Can you work these out from the model? Positions are in its coordinate system, mm. Coordinates: 2 decimals unless noted, no trailing zeros. Loops run counter-clockwise (first coordinate to the right, second up) from the corner with the lowest first, then second, coordinate; pieces in that order, holes last. Notation, with made-up numbers: M 37.25,40 L 60.25,40 A24 cw 60.25,55 Z; hole C -29.75,-24 d7. An arc over 180 degrees is marked long. Return JSON: item names as keys, results as strings. Group by question number.
Autodesk Inventor part; units mm, degrees
ref_plane "YZ Plane" through (0, 0, 0) normal (1, 0, 0) x (0, 1, 0)
ref_plane "XZ Plane" through (0, 0, 0) normal (0, 1, 0) x (-1, 0, 0)
ref_plane "XY Plane" through (0, 0, 0) normal (0, 0, 1) x (1, 0, 0)
sketch "Sketch1" plane through (0, 0, 0) normal (0, 0, 1) x (1, 0, 0)
  line L0 (-88.9, 80.5892) -> (-12.7, 80.5892) construction
  line L1 (-12.7, 80.5892) -> (-12.7, 10.7392) construction
  line L2 (-12.7, 10.7392) -> (-88.9, 10.7392) construction
  line L3 (-88.9, 10.7392) -> (-88.9, 80.5892) construction
  line L4 (-88.9, 80.5892) -> (-88.9, 97.6783) construction
  line L5 (-88.9, 80.5892) -> (-101.6, 80.5892) construction
  line L6 (-101.6, 95.25) -> (-101.6, -6.35)
  line L7 (-12.7, 10.7392) -> (-12.7, -6.35) construction
  line L8 (0, -6.35) -> (-101.6, -6.35)
  line L9 (-12.7, 10.7392) -> (0, 10.7392) construction
  line L10 (0, 95.25) -> (0, -6.35)
  circle A0 centre (-12.7, 80.5892) radius 3.325
  circle A1 centre (-12.7, 10.7392) radius 3.325
  circle A2 centre (-88.9, 10.7392) radius 3.325
  circle A3 centre (-88.9, 80.5892) radius 3.325
  circle A4 centre (-63.3, 45.15) radius 2.1 construction
  circle A5 centre (-63.3, 20.15) radius 2.1 construction
  circle A6 centre (-38.3, 45.15) radius 2.1 construction
  circle A7 centre (-38.3, 20.15) radius 2.1 construction
  circle A8 centre (-63.3, 45.15) radius 4.7625
  circle A9 centre (-38.3, 45.15) radius 2.1 construction
  circle A10 centre (-38.3, 45.15) radius 4.7625
  circle A11 centre (-63.3, 20.15) radius 2.1 construction
  circle A12 centre (-63.3, 20.15) radius 4.7625
  circle A13 centre (-38.3, 20.15) radius 2.1 construction
  circle A14 centre (-38.3, 20.15) radius 4.7625
  line L11 (0, 95.25) -> (-101.6, 95.25) construction
  line L12 (-22.6, 156.65) -> (-79, 156.65) construction
  line L13 (-79, 156.65) -> (-79, 100.25) construction
  line L14 (-79, 100.25) -> (-22.6, 100.25) construction
  line L15 (-22.6, 100.25) -> (-22.6, 156.65) construction
  line L16 (-22.6, 128.45) -> (-79, 128.45) construction
  line L17 (-113.7839, 128.45) -> (12.1839, 128.45) construction
  line L18 (-27.23, 152.02) -> (-74.37, 152.02) construction
  line L19 (-74.37, 152.02) -> (-74.37, 104.88) construction
  line L20 (-74.37, 104.88) -> (-27.23, 104.88) construction
  line L21 (-27.23, 104.88) -> (-27.23, 152.02) construction
  line L22 (-27.23, 152.02) -> (-22.6, 152.02) construction
  line L23 (-27.23, 152.02) -> (-27.23, 156.65) construction
  line L24 (-74.37, 104.88) -> (-79, 104.88) construction
  line L25 (-74.37, 104.88) -> (-74.37, 100.25) construction
  circle A15 centre (-27.23, 152.02) radius 2.6
  circle A16 centre (-27.23, 104.88) radius 2.6
  circle A17 centre (-74.37, 104.88) radius 2.6
  circle A18 centre (-74.37, 152.02) radius 2.6
  circle A19 centre (-50.8, 128.45) radius 19.15
  circle A20 centre (-50.8, 128.45) radius 11.08 construction
  circle A21 centre (-50.8, 128.45) radius 13 construction
  line L26 (-50.8, -6.35) -> (-50.8, 203.8417) construction
  circle A22 centre (-74.37, 104.88) radius 13 construction
  circle A23 centre (-27.23, 104.88) radius 13 construction
  circle A24 centre (-74.37, 104.88) radius 11.08 construction
  circle A25 centre (-27.23, 104.88) radius 11.08 construction
  line L27 (-79, 157.1) -> (-101.6, 95.25)
  line L28 (0, 95.25) -> (-22.6, 157.1)
  line L29 (0, 0) -> (-101.6, 0)
  line L30 (-79, 157.1) -> (-22.6, 157.1)
  line L31 (-63.3, 45.15) -> (-38.3, 45.15) construction
  line L32 (-38.3, 45.15) -> (-38.3, 20.15) construction
  line L33 (-38.3, 20.15) -> (-63.3, 20.15) construction
  line L34 (-63.3, 20.15) -> (-63.3, 45.15) construction
  line L35 (0, 95.25) -> (0, 157.1)
  line L36 (0, 157.1) -> (-22.6, 157.1)
  point P0 (-39.7703, 127.3952)
  point P1 (-39.7703, 127.3951)
  point P2 (-50.8, 128.45)
  dimension "d0" = 6.65
  dimension "d1" = 6.65
  dimension "d2" = 6.65
  dimension "d3" = 6.65
  dimension "d4" = 69.85
  dimension "d5" = 76.2
  dimension "d6" = 9.525
  dimension "d7" = 9.525
  dimension "d8" = 9.525
  dimension "d9" = 9.525
  dimension "d10" = 101.6
  dimension "d12" = 56.4
  dimension "d13" = 56.4
  dimension "d14" = 0
  dimension "d15" = 47.14
  dimension "d16" = 47.14
  dimension "d17" = 5.2
  dimension "d18" = 5.2
  dimension "d19" = 5.2
  dimension "d20" = 5.2
  dimension "d21" = 38.3
  dimension "d22" = 22.16
  dimension "d23" = 26
  dimension "d24" = 28.2
  dimension "d25" = 50.8
  dimension "d26" = 5
  dimension "d27" = 95.25
  dimension "d28" = 26
  dimension "d29" = 26
  dimension "d30" = 22.16
  dimension "d31" = 22.16
  dimension "d34" = 0.45
  dimension "d36" = 25
  dimension "d37" = 25
  dimension "d38" = 26.5
extrude "Extrusion1" add sketch "Sketch1" against normal blind 3.175 contours L27 L30 L28 L10 L29 L6 | L36 L35 L28
fillet "Fillet1" radius 2 3 edges at (-79, 157.1, -1.5875) (-101.6, 95.25, -1.5875) (0, 157.1, -1.5875)
sketch "Sketch2" plane through (0, 0, -3.175) normal (0, 0, -1) x (-1, 0, 0)
  line L0 (0, 157.1) -> (20, 157.1) construction
  line L1 (20, 157.1) -> (20, 102.1) construction
  line L2 (20, 102.1) -> (0, 102.1) construction
  line L3 (0, 102.1) -> (0, 157.1) construction
  line L4 (77.6015, 157.1) -> (2, 157.1) construction
  line L5 (0, 155.1) -> (0, 0) construction
  line L6 (10, 102.1) -> (10, 157.1) construction
  line L7 (2, 157.1) -> (77.6015, 157.1) construction
  circle A0 centre (10, 142.1) radius 2.6
  circle A1 centre (10, 117.1) radius 2.6
  dimension "d39" = 20
  dimension "d40" = 55
  dimension "d41" = 5.2
  dimension "d42" = 5.2
  dimension "d43" = 15
  dimension "d44" = 15
extrude "Extrusion2" cut sketch "Sketch2" against normal up to next
fillet "Fillet2" radius 3.175 2 edges at (0, 0, -1.5875) (-101.6, 0, -1.5875)
equation "\"d0\" = d3"
equation "\"d1\" = d3"
equation "\"d2\" = d3"
equation "\"d7\" = d6"
equation "\"d8\" = d6"
equation "\"d9\" = d6"
equation "\"d16\" = d15"
equation "\"d18\" = d17"
equation "\"d19\" = d17"
equation "\"d20\" = d17"
equation "\"d24\" = 0.5 * d12"
equation "\"d44\" = d43"
properties part number "X Axis Belt Motor Frame Machined"
1) For pin 1 (3 mm diameter, centred on x = -27.23, y = 152.02, fed in from +Z), with a flat end and sliding along its axis, tell me the tip position at first contact or that it passes through.
2) Suppose I cut it at A-A, the plane x = -27.23. List the corners of the cut face in (y, z) for me (3 decimals), then the cut area to 3 significant figures.
3) If we mould it in two halves opening along X, with no side actions, what happens to faces 1 (the face through (-9.662, 144.678, -1.61)), 2 (the face through (-90.325, 126.106, -1.565)), 3 (the face through (-27.568, 154.598, -1.565)), 4 (the face through (-52, 80, 0))? For each: +X half, -X half, draft (parallel to the pull), parting line (faces both ways), or undercut.
4) Suppose I cut it at D-D, the plane y = 128.45. List the corners of the cut face in (x, z) for me (3 decimals), then the cut area to 3 significant figures.
5) Suppose I cut it at B-B, the plane y = 45.15. List the corners of the cut face in (x, z) for me (1 decimal), then the cut area to 3 significant figures.
6) Suppose I cut it at C-C, the plane x = -38.3. List the corners of the cut face in (y, z) for me (1 decimal), then the cut area to 3 significant figures.
7) If I drill on line 1 (X direction, y = 81, z = -1.1); line 2 (Y direction, x = -27.23, z = -1.9); line 3 (Y direction, x = -10.5, z = -0.9), over which ranges is the centre line in solid material (lowest first)? Write a range as from..to.
Returned:
{
 "1": {"pin 1": "passes through"},
 "2": {"outline": "M 0,-3.175 L 102.28,-3.175 L 102.28,0 L 0,0 Z; M 107.48,-3.175 L 149.42,-3.175 L 149.42,0 L 107.48,0 Z; M 154.62,-3.175 L 157.1,-3.175 L 157.1,0 L 154.62,0 Z", "area": "466 mm²"},
 "3": {"face 1": "undercut", "face 2": "-X half", "face 3": "undercut", "face 4": "draft"},
 "4": {"outline": "M -89.469,-3.175 L -69.95,-3.175 L -69.95,0 L -89.469,0 Z; M -31.65,-3.175 L 0,-3.175 L 0,0 L -31.65,0 Z", "area": "162 mm²"},
 "5": {"outline": "M -101.6,-3.2 L -68.1,-3.2 L -68.1,0 L -101.6,0 Z; M -58.5,-3.2 L -43.1,-3.2 L -43.1,0 L -58.5,0 Z; M -33.5,-3.2 L 0,-3.2 L 0,0 L -33.5,0 Z", "area": "262 mm²"},
 "6": {"outline": "M 0,-3.2 L 15.4,-3.2 L 15.4,0 L 0,0 Z; M 24.9,-3.2 L 40.4,-3.2 L 40.4,0 L 24.9,0 Z; M 49.9,-3.2 L 113.9,-3.2 L 113.9,0 L 49.9,0 Z; M 143,-3.2 L 157.1,-3.2 L 157.1,0 L 143,0 Z", "area": "346 mm²"},
 "7": {"line 1": "x = -101.6..-92.2, -85.6..-16, -9.4..0", "line 2": "y = 0..102.28, 107.48..149.42, 154.62..157.1", "line 3": "y = 0..8.25, 13.23..78.1, 83.08..114.55, 119.65..139.55, 144.65..157.1"}
}
